Part model, mm, in its own coordinate system. Round coordinates to 2 decimals unless told otherwise and drop trailing zeros. Order: outer loops, then holes, each group sorted by start corner. A loop starts at its lowest first (then second) coordinate and runs counter-clockwise, first axis right, second up. Notation, with made-up numbers: (-13.5, -18) - (-4.5, -18) arc R13 cw to (-4.5, -14) - close; hole circle Ø3 at (-24.5, 39.5). An arc over 180 degrees is marked (long way). Return JSON: item names as keys, results as strings. Group by question number.
Item 1: Probe probe 1 along Y at (x, z) = (-232.5, -158.75) (3 decimals); probe 2 along Z at (x, y) = (-233.4, 32); probe 3 along Y at (x, z) = (-230.9, -176) (3 decimals). List the from-to ranges inside material, lowest first.
Item 2: Two-plate mould, pull along Y, no slides. Class faces 1 (the face through (-232.6, 122.44, -150.75)), 2 (the face through (-232.54, 106.84, -156.16)), 3 (the face through (-232.6, 1.81, -204.99)): released by +Y, released by -Y, zero draft, split by the parting line, or undercut.
Item 3: Saw through at A-A on y = 9. List the corners of the cut face in (x, z), and give its area (3 significant figures).
Item 4: Saw through at B-B on z = -158.75. State how many separate pieces and enclosed holes the cut face has, and give its area (3 significant figures).
```python
from build123d import *

# Parameters (mm, degrees)
SKETCH1_R           = 3.2639
BOSS_EXTRUDE1_DEPTH = 4.7625
FILLET1_R           = 6.35


with BuildPart() as part:
    # Sketch1 → Boss-Extrude1 (new body)
    with BuildSketch(Plane(origin=(-230.1875, 0, 0), x_dir=(0, 0, -1), z_dir=(1, 0, 0))):
        Polygon((130.7, 0), (206.9, 0), (206.9, 47.625), (187.85, 123.825), (149.75, 123.825), (130.7, 47.625), align=None)
        with Locations((194.2, 29.1)):
            Circle(SKETCH1_R, mode=Mode.SUBTRACT)
        with Locations((158.75, 108.825000028)):
            Circle(SKETCH1_R, mode=Mode.SUBTRACT)
        with Locations((178.85, 108.825000028)):
            Circle(SKETCH1_R, mode=Mode.SUBTRACT)
        with Locations((178.85, 62.625)):
            Circle(SKETCH1_R, mode=Mode.SUBTRACT)
        with Locations((158.75, 62.625)):
            Circle(SKETCH1_R, mode=Mode.SUBTRACT)
        with Locations((143.4, 29.1)):
            Circle(SKETCH1_R, mode=Mode.SUBTRACT)
        with Locations((143.4, 9)):
            Circle(SKETCH1_R, mode=Mode.SUBTRACT)
        with Locations((194.2, 9)):
            Circle(SKETCH1_R, mode=Mode.SUBTRACT)
    extrude(amount=-BOSS_EXTRUDE1_DEPTH)

    # Fillet1
    fillet1_edges = [part.edges().sort_by_distance(p)[0] for p in [
        (-232.56875, 0, -130.7),
        (-232.56875, 0, -206.9),
        (-232.56875, 47.625, -206.9),
        (-232.56875, 47.625, -130.7),
        (-232.56875, 123.825, -187.85),
        (-232.56875, 123.825, -149.75),
    ]]
    fillet(fillet1_edges, radius=FILLET1_R)


solid = part.part
```
Filled in:
{
 "1": {"probe 1": "y = 0 to 59.361, 65.889 to 105.561, 112.089 to 123.825", "probe 2": "z = -206.9 to -195.7, -192.7 to -144.9, -141.9 to -130.7", "probe 3": "y = 0 to 61.034, 64.216 to 107.234, 110.416 to 123.825"},
 "2": {"face 1": "released by +Y", "face 2": "undercut", "face 3": "released by -Y"},
 "3": {"outline": "(-234.95, -206.9) - (-230.19, -206.9) - (-230.19, -197.46) - (-234.95, -197.46) - close; (-234.95, -190.94) - (-230.19, -190.94) - (-230.19, -146.66) - (-234.95, -146.66) - close; (-234.95, -140.14) - (-230.19, -140.14) - (-230.19, -130.7) - (-234.95, -130.7) - close", "area": "301 mm^2"},
 "4": {"separate pieces": "3", "enclosed holes": "0", "area": "528 mm^2"}
}
